from build123d import *

# Parameters (mm, degrees)
BOSS_EXTRUDE1_DEPTH = 25
SKETCH2_R           = 1.75
BOSS_EXTRUDE2_DEPTH = 2
FILLET1_R           = 3


with BuildPart() as part:
    # Sketch1 → Boss-Extrude1 (new, symmetric)
    with BuildSketch(Plane.XY):
        Polygon((0, 0), (15, 0), (15, 6.994614872), align=None)
    extrude(amount=BOSS_EXTRUDE1_DEPTH, both=True)

    # Sketch2 → Boss-Extrude2 (add)
    with BuildSketch(Plane.XY.offset(25)):
        Polygon((15, 0), (15, 27.5), (11, 27.5), (0, 0), align=None)
        with Locations((12, 23.5)):
            Circle(SKETCH2_R, mode=Mode.SUBTRACT)
        with Locations((12, 17.5)):
            Circle(SKETCH2_R, mode=Mode.SUBTRACT)
    boss_extrude2 = extrude(amount=BOSS_EXTRUDE2_DEPTH)

    # Mirror1: Boss-Extrude2 across plane
    add(boss_extrude2.mirror(Plane.XY))

    # Fillet1
    fillet1_edges = [part.edges().sort_by_distance(p)[0] for p in [
        (15, 0, 0),
    ]]
    fillet(fillet1_edges, radius=FILLET1_R)


solid = part.part
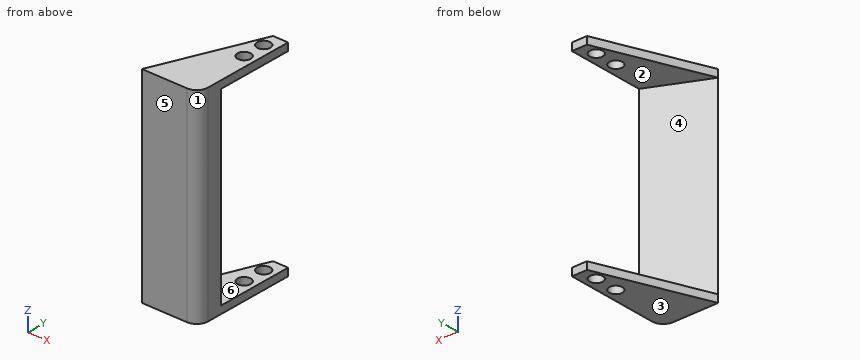
Geometry: final body of the model. Coordinates: model frame, mm. Face numbers are marked on the shaded views. A direction names the side the tool comes from. Coordinates: 2 decimals unless noted, no trailing zeros. Loops run counter-clockwise (first coordinate to the right, second up) from the corner with the lowest first, then second, coordinate; pieces in that order, holes last. Notation, with made-up numbers: (76.5, 23) - (96.5, 23) arc R7 cw to (96.5, 29) - close; hole circle Ø6 at (75, -38.75). An arc over 180 degrees is marked (long way). Put each result on its own line as item: value. Start each with the question number.
Q1. Cut plane D-D, the plane x = 2.75. Return loops of the section in (y, z) (3 decimals).
Q2. Set-up query: the marked faces 1 and 2. Return all of +Z, -Z, +X, -X, +Y, -Y with unobstructed straight access to the full face (end or side cutting, diameter ignored); none if empty.
Q3. Cut plane A-A, the plane y = 21.25. Return loops of the section in (x, z).
Q4. Cut plane C-C, the plane x = 12.75. Return loops of the section in (y, z).
Q5. Pull-direction query (Z, two-part tool) for the marked faces 3, 4, 5 and 6; classes: released by +Z, released by -Z, zero draft, split by the parting line, or undercut.
Q6. Line query: line 1 (Y direction, x = 12, z = -26.2); line 2 (Z direction, x = 5.5, y = 10.25); line 3 (Y direction, x = 11, z = 15.5). Output: solid intervals per line, ascending.
Q7. Cut plane B-B, the plane y = 17.5. Return loops of the section in (x, z), and give its area (3 significant figures).
Filled sheet:
1. outline: (0, -27) - (6.875, -27) - (6.875, -25) - (1.282, -25) - (1.282, 25) - (6.875, 25) - (6.875, 27) - (0, 27) - close
2. face 1: +Z, -Z, +X, -Y
2. face 2: -X, +Y
3. outline: (8.5, -27) - (15, -27) - (15, -25) - (8.5, -25) - close; (8.5, 25) - (15, 25) - (15, 27) - (8.5, 27) - close
4. outline: (0.1, -27) - (15.92, -27) - (15.92, -25) - (5.95, -25) - (5.95, 25) - (15.92, 25) - (15.92, 27) - (0.1, 27) - close; (19.08, -27) - (21.92, -27) - (21.92, -25) - (19.08, -25) - close; (19.08, 25) - (21.92, 25) - (21.92, 27) - (19.08, 27) - close; (25.08, -27) - (27.5, -27) - (27.5, -25) - (25.08, -25) - close; (25.08, 25) - (27.5, 25) - (27.5, 27) - (25.08, 27) - close
5. face 3: released by -Z
5. face 4: undercut
5. face 5: zero draft
5. face 6: undercut
6. line 1: 0 to 15.75, 19.25 to 21.75, 25.25 to 27.5
6. line 2: -27 to -25, 25 to 27
6. line 3: 0 to 5.13
7. outline: (7, -27) - (10.25, -27) - (10.25, -25) - (7, -25) - close; (7, 25) - (10.25, 25) - (10.25, 27) - (7, 27) - close; (13.75, -27) - (15, -27) - (15, -25) - (13.75, -25) - close; (13.75, 25) - (15, 25) - (15, 27) - (13.75, 27) - close
7. area: 18.0 mm²
